```python
from build123d import *

# Parameters (mm, degrees)
SKETCH1_R           = 4
BOSS_EXTRUDE1_DEPTH = 95
SKETCH1_3_R         = 6
SKETCH1_3_R_2       = 4
BOSS_EXTRUDE2_DEPTH = 50.5


with BuildPart() as part:
    # Sketch1 → Boss-Extrude1 (new, symmetric)
    with BuildSketch(Plane(origin=(0, 0, 0), x_dir=(1, 0, 0), z_dir=(0, 1, 0))):
        with Locations(Location((0, 0, 0), (0, 0, 270))):
            Circle(SKETCH1_R)
    extrude(amount=BOSS_EXTRUDE1_DEPTH, both=True)

    # Sketch1_3 → Boss-Extrude2 (add, symmetric)
    with BuildSketch(Plane(origin=(0, 0, 0), x_dir=(1, 0, 0), z_dir=(0, 1, 0))):
        with Locations(Location((0, 0, 0), (0, 0, 270))):
            Circle(SKETCH1_3_R)
        with Locations(Location((0, 0, 0), (0, 0, 270))):
            Circle(SKETCH1_3_R_2, mode=Mode.SUBTRACT)
    extrude(amount=BOSS_EXTRUDE2_DEPTH, both=True)


solid = part.part
```
The model under review builds one solid part; all positions refer to its coordinate system, in mm. A direction names the side the tool comes from. Give positions to 0.01 mm unless a question says otherwise; leave off trailing zeros. Write each loop counter-clockwise with the first axis right and the second up, starting at its lowest first coordinate (ties: lowest second). Pieces come first, ordered by that corner, then holes. Notation, with made-up numbers: (17.25, 64.5) -> (22.25, 64.5) arc R17 ccw to (22.25, 85.5) -> close; hole circle Ø7 at (18, 37.5). An arc over 180 degrees is marked (long way). Answer in a Markdown table with one row per item.
1) Add section B-B on z = 0. State the section outline as (x, y) points, plus the area to 3 significant figures.
Worked answers:
| item | result |
|---|---|
| outline | (-6, -50.5) -> (-4, -50.5) -> (-4, -95) -> (4, -95) -> (4, -50.5) -> (6, -50.5) -> (6, 50.5) -> (4, 50.5) -> (4, 95) -> (-4, 95) -> (-4, 50.5) -> (-6, 50.5) -> close |
| area | 1,920 mm² |
2) Add section A-A on x = 0. State the section outline as (y, z) points, plus the area to 3 significant figures.
Worked answers:
| item | result |
|---|---|
| outline | (-95, -4) -> (-50.5, -4) -> (-50.5, -6) -> (50.5, -6) -> (50.5, -4) -> (95, -4) -> (95, 4) -> (50.5, 4) -> (50.5, 6) -> (-50.5, 6) -> (-50.5, 4) -> (-95, 4) -> close |
| area | 1,920 mm² |
3) For L1, parallel to Y at x = 4.5, z = 0; L2, parallel to X at y = -44.5, z = 4.5; L3, parallel to X at y = -7, z = -0.5, list the stretches that pass through material, from the lowest coordinate up. Write a range as [from, to].
Worked answers:
| item | result |
|---|---|
| L1 | [-50.5, 50.5] |
| L2 | [-3.97, 3.97] |
| L3 | [-5.98, 5.98] |
4) Clearance check with flat-ended pins moving along their axes: P1, Ø4, axis at y = -53.5, z = -4, coming from the -X side; P2, Ø1.5, axis at x = -3, y = 68, coming from the -Z side; P3, Ø5, axis at y = -55, z = -2, coming from the -X side. State where each tip first meets the part, or that it passes through.
Worked answers:
| item | result |
|---|---|
| P1 | x = -3.46 |
| P2 | z = -3.31 |
| P3 | x = -4 |
5) Add section D-D on y = 27. State the section outline as (x, z) points.
Worked answers:
| item | result |
|---|---|
| outline | circle Ø12 at (0, 0) |
6) Add section C-C on y = 76. State the section outline as (x, z) points.
Worked answers:
| item | result |
|---|---|
| outline | circle Ø8 at (0, 0) |
7) Tool access review of faces 1 (the flat face through (-3.92, -50.5, -1.42)), 2 (the cylindrical face through (-3.905, 73.062, -0.867)), 3 (the cylindrical face through (1.802, 0.707, 5.723)): name each direction out of +Z, -Z, +X, -X, +Y, -Y from which nothing blocks a thin tool from reaching the whole face with its end or side.
Worked answers:
| item | result |
|---|---|
| face 1 | -Y |
| face 2 | +Y |
| face 3 | +Y, -Y |
